Part print with two shaded views. Sizes in mm from the minimum x, y, z corner. Coordinates: 2 decimals unless noted, no trailing zeros. Loops run counter-clockwise (first coordinate to the right, second up) from the corner with the lowest first, then second, coordinate; pieces in that order, holes last.
(1) Wall check: L1, parallel to X at y = 0.7, z = 19; L2, parallel to X at y = 0.3, z = 31 (1 decimal); L3, parallel to Z at x = 49, y = 0.7 (1 decimal). Give the ranges that are in metal, low to high.
(2) Slice it at C-C (z = 9). Give the cut face in (x, y) (1 decimal).
(3) Slice it at D-D (y = 0.6). Give the cut face in (x, z) (1 decimal), and give its area (3 significant figures).
(4) Slice it at A-A (x = 28). Give the cut face in (y, z).
(5) Slice it at B-B (z = 39). Give the cut face in (x, y) (1 decimal).
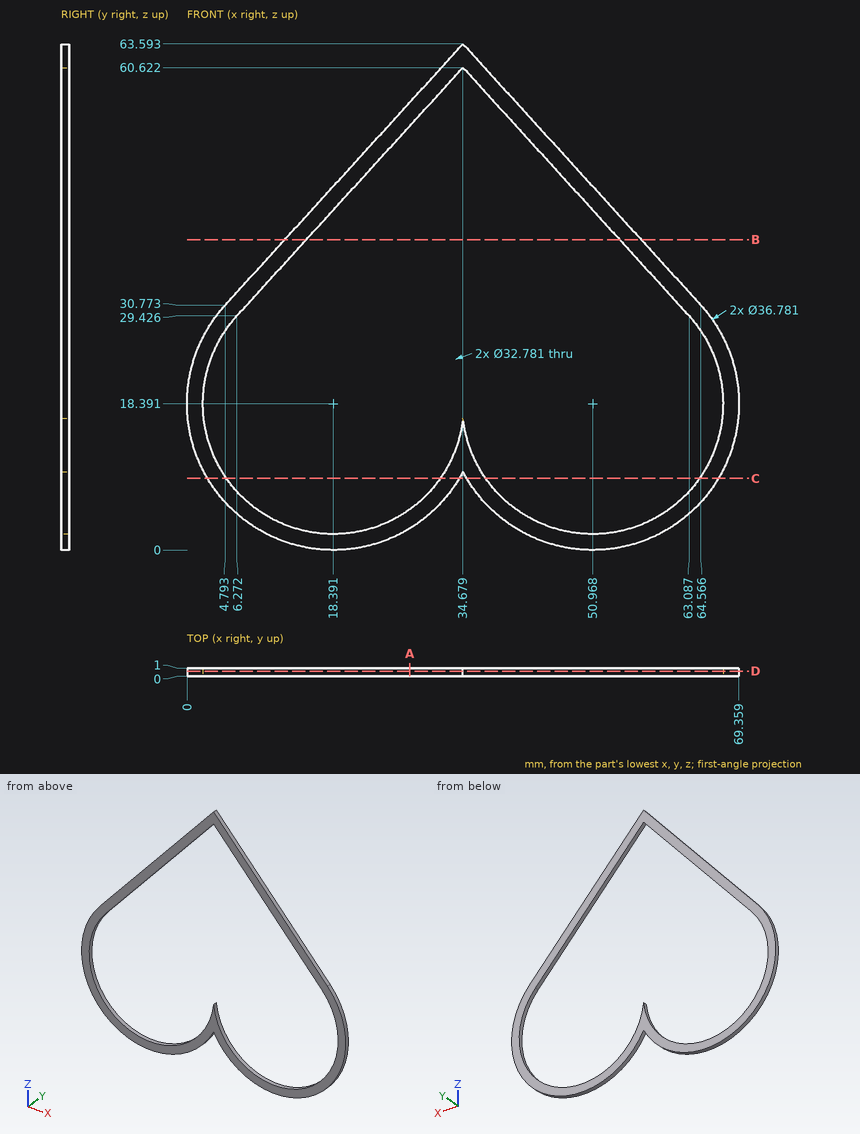
Response values:
1. L1: x = 0.01 to 2.01, 67.35 to 69.35
1. L2: x = 5 to 7.7, 61.7 to 64.4
1. L3: z = 0.1 to 2.1, 44.9 to 47.9
2. outline: (2.6, 0) - (5, 0) - (5, 1) - (2.6, 1) - close; (31.8, 0) - (34.2, 0) - (34.2, 1) - (31.8, 1) - close; (35.2, 0) - (37.5, 0) - (37.5, 1) - (35.2, 1) - close; (64.4, 0) - (66.8, 0) - (66.8, 1) - (64.4, 1) - close
3. outline: (4.8, 30.8) arc R18.4 ccw (long way) to (34.7, 9.9) arc R18.4 ccw (long way) to (64.6, 30.8) - (34.7, 63.6) - close; hole (6.3, 29.4) arc R16.4 ccw (long way) to (34.7, 16.6) arc R16.4 ccw (long way) to (63.1, 29.4) - (34.7, 60.6) - close
3. area: 419 mm2
4. outline: (0, 2.71) - (1, 2.71) - (1, 5.11) - (0, 5.11) - close; (0, 53.29) - (1, 53.29) - (1, 56.26) - (0, 56.26) - close
5. outline: (12.3, 0) - (15, 0) - (15, 1) - (12.3, 1) - close; (54.4, 0) - (57.1, 0) - (57.1, 1) - (54.4, 1) - close
